from build123d import *

# Parameters (mm, degrees)
SKETCH1_W           = 150
SKETCH1_H           = 48
SKETCH1_R           = 3.1
BOSS_EXTRUDE1_DEPTH = 5
BOSS_EXTRUDE2_DEPTH = 20
BOSS_EXTRUDE3_DEPTH = 25
BOSS_EXTRUDE4_START = -150
BOSS_EXTRUDE4_DEPTH = 25
BOSS_EXTRUDE5_START = -75
BOSS_EXTRUDE5_DEPTH = 32.5
FILLET5_SIZE        = 10
FILLET5_SIZE_2      = 4
FILLET6_SIZE        = 10
FILLET6_SIZE_2      = 4


with BuildPart() as part:
    # Sketch1 → Boss-Extrude1 (new body)
    with BuildSketch(Plane.XY):
        with Locations((0, 24)):
            Rectangle(SKETCH1_W, SKETCH1_H)
        with Locations((-41, 10)):
            Circle(SKETCH1_R, mode=Mode.SUBTRACT)
        with Locations((41, 10)):
            Circle(SKETCH1_R, mode=Mode.SUBTRACT)
    extrude(amount=BOSS_EXTRUDE1_DEPTH)

    # Sketch2 → Boss-Extrude2 (add)
    with BuildSketch(Plane.XY):
        with BuildLine():
            Line((-75, 5), (-75, 0))
            Line((-75, 0), (75, 0))
            Line((75, 0), (75, 5))
            Line((75, 5), (48.5, 5))
            add(Edge.make_bspline(
                [(33.5, 5), (36.476810307, 4.895138539), (41.670990079, -0.895128503), (44.181209535, 4.895118466), (48.5, 5)],
                knots=[0, 0, 0, 0, 0.5, 1, 1, 1, 1], degree=3))
            Line((33.5, 5), (-33.5, 5))
            add(Edge.make_bspline(
                [(-48.5, 5), (-45.523189693, 4.895138539), (-40.329009921, -0.895128503), (-37.818790465, 4.895118466), (-33.5, 5)],
                knots=[0, 0, 0, 0, 0.5, 1, 1, 1, 1], degree=3))
            Line((-48.5, 5), (-75, 5))
        make_face()
    extrude(amount=BOSS_EXTRUDE2_DEPTH)

    # Sketch4 → Boss-Extrude3 (add)
    with BuildSketch(Plane.ZY.offset(75)):
        Polygon((5, 5), (12.5, 5), (5, 15), align=None)
    extrude(amount=-BOSS_EXTRUDE3_DEPTH)

    # Sketch4<2> → Boss-Extrude4 (add)
    with BuildSketch(Plane.ZY.offset(75).offset(BOSS_EXTRUDE4_START)):
        Polygon((5, 5), (12.5, 5), (5, 15), align=None)
    extrude(amount=BOSS_EXTRUDE4_DEPTH)

    # Sketch4<3> → Boss-Extrude5 (add, symmetric)
    with BuildSketch(Plane.ZY.offset(75).offset(BOSS_EXTRUDE5_START)):
        Polygon((5, 5), (12.5, 5), (5, 15), align=None)
    extrude(amount=BOSS_EXTRUDE5_DEPTH, both=True)

    # Fillet5
    # an asymmetric fillet: 10, 4 mm, written as the material it takes off along each edge
    with BuildSketch(Plane(origin=(-75, 0, 45), x_dir=(1, 0, 0), z_dir=(0, 0, -1))) as fillet5_piece_1:
        with BuildLine():
            Bezier((FILLET5_SIZE, 0), (0, 0), (0, -FILLET5_SIZE_2), weights=[1, 0.707106781, 1])
            Line((0, -FILLET5_SIZE_2), (0, 0))
            Line((0, 0), (FILLET5_SIZE, 0))
        make_face()
    extrude(amount=70, mode=Mode.SUBTRACT)

    # Fillet6
    # an asymmetric fillet: 10, 4 mm, written as the material it takes off along each edge
    with BuildSketch(Plane(origin=(75, 0, -25), x_dir=(-1, 0, 0), z_dir=(0, 0, 1))) as fillet6_piece_1:
        with BuildLine():
            Bezier((FILLET6_SIZE, 0), (0, 0), (0, -FILLET6_SIZE_2), weights=[1, 0.707106781, 1])
            Line((0, -FILLET6_SIZE_2), (0, 0))
            Line((0, 0), (FILLET6_SIZE, 0))
        make_face()
    extrude(amount=70, mode=Mode.SUBTRACT)


solid = part.part
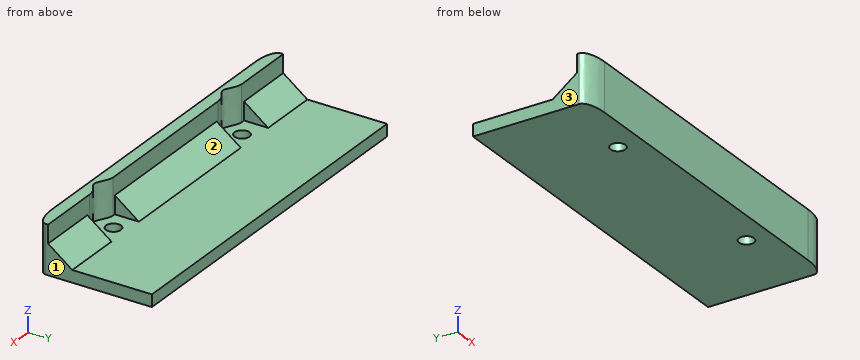
Can you work these out from the model? Positions are in its coordinate system, mm. Face numbers are marked on the shaded views. Coordinates: 2 decimals unless noted, no trailing zeros. Loops run counter-clockwise (first coordinate to the right, second up) from the corner with the lowest first, then second, coordinate; pieces in that order, holes last. Notation, with made-up numbers: M 74.5,8.25 L 131.5,8.25 A20 ccw 131.5,34.25 Z; hole C -29,29.5 d5. An arc over 180 degrees is marked long. Return JSON: item names as keys, results as strings. Group by question number.
Item 1: Imagine slicing it at A-A (y = 10). Please give me the cut outline in (x, z).
Item 2: I'm going to push flat-ended pins straight in: pin 1 Ø1 at (y, z) = (19, 6) entering from -X; pin 2 Ø5 at (x, z) = (48.5, 17.5) entering from -Y; pin 3 Ø4.5 at (x, z) = (-10.5, 11.5) entering from +Y; pin 4 Ø8 at (x, z) = (40.5, 10) entering from +Y. Where does each tip first touch, or does it pass through?
Item 3: Imagine slicing it at C-C (y = 27). Please give me the cut outline in (x, z), and give its area (3 significant figures).
Item 4: Imagine slicing it at B-B (x = 62). Please give me the cut outline in (y, z), and give its area (4 significant figures).
Item 5: If I drill on L1, parallel to Y at x = -41, z = 3.15; L2, parallel to Z at x = 33.5, y = 39; L3, parallel to Y at x = -65.5, z = 18.5 (3 decimals), over which ranges is the centre line in solid material (lowest first)? Write a range as from..to.
Item 6: Thinking about a two-plate mould opening in X: for the marked faces 1, 2 and 3, which applies, released by +X, released by -X, zero draft, split by the parting line, or undercut?
Verdict:
{
 "1": {"outline": "M -75,0 L -44.1,0 L -44.1,5 L -50,5 L -50,8.75 L -75,8.75 Z; M -37.9,0 L 37.9,0 L 37.9,5 L 32.5,5 L 32.5,8.75 L -32.5,8.75 L -32.5,5 L -37.9,5 Z; M 44.1,0 L 75,0 L 75,8.75 L 50,8.75 L 50,5 L 44.1,5 Z"},
 "2": {"pin 1": "passes through", "pin 2": "stops at y = 0", "pin 3": "stops at y = 9.33", "pin 4": "stops at y = 4.09"},
 "3": {"outline": "M -75,0 L 75,0 L 75,5 L -75,5 Z", "area": "750 mm^2"},
 "4": {"outline": "M 0,0 L 48,0 L 48,5 L 15,5 L 5,12.5 L 5,20 L 0,20 Z", "area": "352.5 mm^2"},
 "5": {"L1": "y = 0..6.9, 13.1..48", "L2": "z = 0..5", "L3": "y = 0.005..5"},
 "6": {"face 1": "released by +X", "face 2": "zero draft", "face 3": "released by -X"}
}
